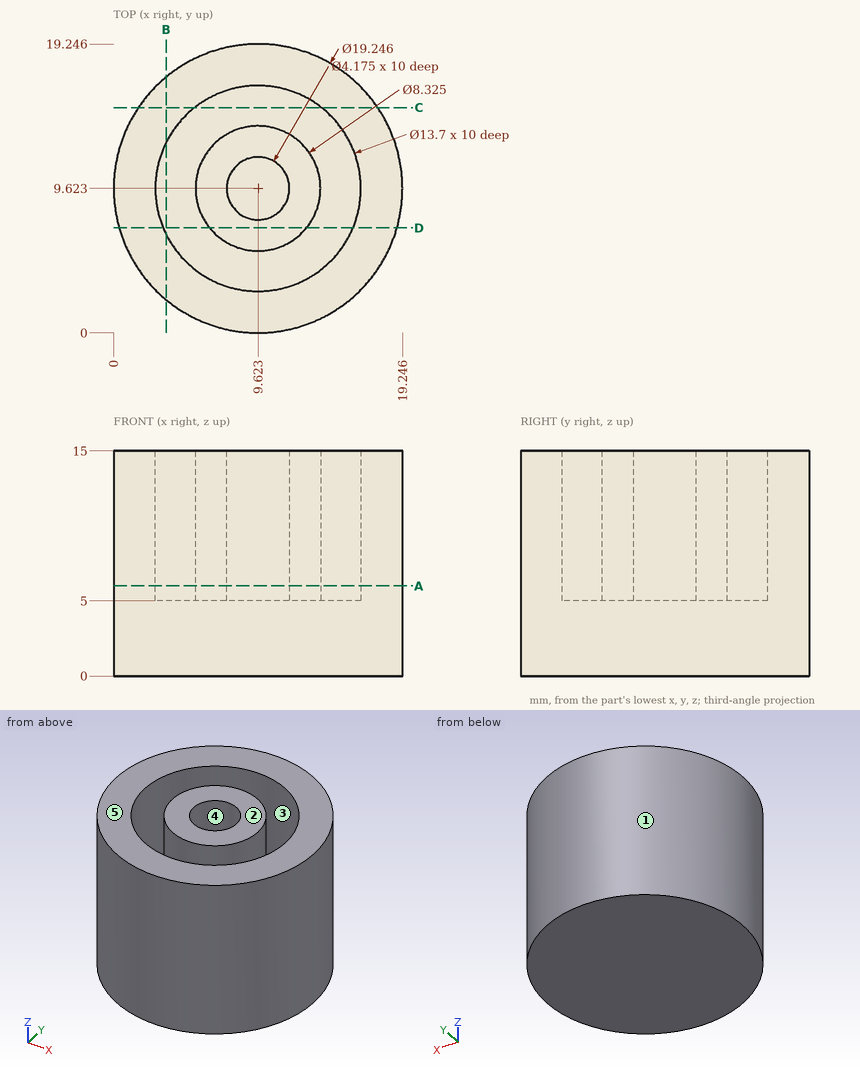
Source: three-view drawing plus pictorial views. Frame: mm from the lowest corner of the part. A direction names the side the tool comes from. Round coordinates to 2 decimals unless told otherwise and drop trailing zeros. Write each loop counter-clockwise with the first axis right and the second up, starting at its lowest first coordinate (ties: lowest second). Pieces come first, ordered by that corner, then holes. Notation, with made-up numbers: (34.5, -24.5) -> (65.5, -24.5) arc R15 ccw to (65.5, -8.5) -> close; hole circle Ø4 at (66.25, 72.5). An arc over 180 degrees is marked (long way). Return JSON: item names as keys, results as strings.
Q1. Section A-A on z = 6. Give the number of separate pieces and of enclosed holes in the cut face, and give its area (3 significant figures).
From the geometry:
{"separate pieces": "2", "enclosed holes": "2", "area": "184 mm2"}
Q2. Ray query, line 1 (Y direction, x = 13.25, z = 8); line 2 (X direction, y = 12.25, z = 7.75); line 3 (Y direction, x = 7.5, z = 12). Return the intervals inside material, ascending.
From the geometry:
{"line 1": "0.71 to 3.81, 7.58 to 11.67, 15.43 to 18.54", "line 2": "0.37 to 3.3, 6.39 to 12.85, 15.95 to 18.88", "line 3": "0.24 to 3.11, 6.04 to 13.2, 16.14 to 19.01"}
Q3. Set-up query: the marked faces 4 and 5. Return all of +Z, -Z, +X, -X, +Y, -Y with unobstructed straight access to the full face (end or side cutting, diameter ignored); none if empty.
From the geometry:
{"face 4": "+Z", "face 5": "+Z, +X, -X, +Y, -Y"}
Q4. Section B-B on x = 3.5. Return the cut outline in (y, z).
From the geometry:
{"outline": "(2.2, 0) -> (17.05, 0) -> (17.05, 15) -> (12.69, 15) -> (12.69, 5) -> (6.55, 5) -> (6.55, 15) -> (2.2, 15) -> close"}
Q5. Section D-D on y = 7. Return the cut outline in (x, z).
From the geometry:
{"outline": "(0.36, 0) -> (18.88, 0) -> (18.88, 15) -> (15.95, 15) -> (15.95, 5) -> (12.86, 5) -> (12.86, 15) -> (6.39, 15) -> (6.39, 5) -> (3.3, 5) -> (3.3, 15) -> (0.36, 15) -> close"}
Q6. Mould query, pull axis X, two halves, no side actions, for the marked faces 1, 2 and 3. Classes: +X half, -X half, draft (parallel to the pull), parting line (faces both ways), or undercut.
From the geometry:
{"face 1": "parting line", "face 2": "draft", "face 3": "undercut"}
Q7. First-contact query: pin 1 Ø5.5 at (x, y) = (9.623, 9.623) entering from +Z; pin 2 Ø1 at (y, z) = (10.5, 2) entering from -X; pin 3 Ø2 at (x, z) = (4.5, 13.5) entering from +Y; pin 4 Ø4 at (y, z) = (17, 6) entering from +X. Flat tips, straight axial feed; report the tip coordinate or a pass-through.
From the geometry:
{"pin 1": "z = 15", "pin 2": "x = 0.01", "pin 3": "y = 18.32", "pin 4": "x = 17.6"}
Q8. Section C-C on y = 15. Return the cut outline in (x, z), and give its area (3 significant figures).
From the geometry:
{"outline": "(1.64, 0) -> (17.6, 0) -> (17.6, 15) -> (13.87, 15) -> (13.87, 5) -> (5.38, 5) -> (5.38, 15) -> (1.64, 15) -> close", "area": "155 mm2"}
